Autodesk Inventor part; units mm, degrees
ref_plane "YZ Plane" through (0, 0, 0) normal (1, 0, 0) x (0, 1, 0)
ref_plane "XZ Plane" through (0, 0, 0) normal (0, 1, 0) x (-1, 0, 0)
ref_plane "XY Plane" through (0, 0, 0) normal (0, 0, 1) x (1, 0, 0)
sketch "Sketch1" plane through (0, 0, 0) normal (0, 1, 0) x (-1, 0, 0)
  line L0 (-6.7, 6.25) -> (6.7, 6.25)
  line L1 (6.7, 6.25) -> (6.7, -6.25)
  line L2 (6.7, -6.25) -> (-6.7, -6.25)
  line L3 (-6.7, -6.25) -> (-6.7, 6.25)
  line L4 (-6.7, 6.25) -> (6.7, -6.25) construction
  line L5 (6.7, 6.25) -> (-6.7, -6.25) construction
  point P0 (0, 0)
  dimension "d0" = 13.4
  dimension "d1" = 12.5
extrude "Extrusion1" add sketch "Sketch1" along normal blind 6.5
sketch "Sketch2" plane through (0, 6.5, 0) normal (0, 1, 0) x (1, 0, 0)
  circle A0 centre (0, 0) radius 3.5
  dimension "d4" = 7
extrude "Extrusion2" add sketch "Sketch2" along normal blind 5
sketch "Sketch3" plane through (0, 11.5, 0) normal (0, 1, 0) x (1, 0, 0)
  circle A0 centre (0, 0) radius 3
  dimension "d7" = 6
extrude "Extrusion3" add sketch "Sketch3" along normal blind 10
sketch "Sketch4" plane through (0, 21.5, 0) normal (0, 1, 0) x (1, 0, 0)
  line L0 (0, -1.5) -> (2.5981, -1.5)
  circle A0 centre (0, 0) radius 3
  line L1 (0, -1.5) -> (-2.5981, -1.5)
  arc A1 (-2.5981, -1.5) -> (2.5981, -1.5) centre (0, 0) ccw
  dimension "d10" = 1.5
extrude "Extrusion4" cut sketch "Sketch4" against normal blind 7 contours L0 A0 L1 picked at (-1.5934, -1.6862)
thread "Thread1"
properties part number "PEC11R-4215F-S0024"
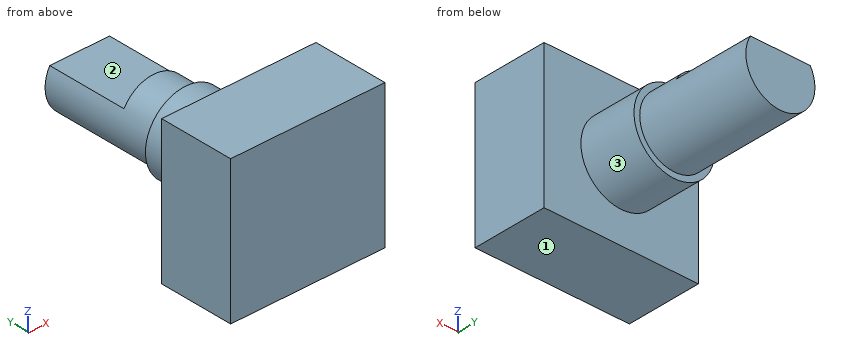
Input: part model. Units: mm. Frame: model coordinates. Face numbers are marked on the shaded views. A direction names the side the tool comes from. Give positions to 0.01 mm unless a question says otherwise; leave off trailing zeros. Loops run counter-clockwise (first coordinate to the right, second up) from the corner with the lowest first, then second, coordinate; pieces in that order, holes last.
1) Contact query for flat-ended pins moving along their axis: pin 1 (5.5 mm diameter, centred on x = 0, y = 17, fed in from +Z); pin 2 (0.5 mm diameter, centred on x = -1, z = 2, fed in from +Y); pin 3 (3 mm diameter, centred on x = -5, y = 12.5, fed in from +Z); pin 4 (1.5 mm diameter, centred on y = 12.5, z = 1, fed in from -X). Output: stop coordinate, or through.
A:
pin 1: stops at z = 3
pin 2: stops at y = 14.5
pin 3: passes through
pin 4: stops at x = -2.99
2) Section query B-B on z = 0. Return the cut outline in (x, y), and give its area (3 significant figures).
A:
outline: (-6.7, 0) - (6.7, 0) - (6.7, 6.5) - (3.5, 6.5) - (3.5, 11.5) - (3, 11.5) - (3, 21.5) - (-3, 21.5) - (-3, 11.5) - (-3.5, 11.5) - (-3.5, 6.5) - (-6.7, 6.5) - close
area: 182 mm2
3) Section query D-D on z = 2.25. Return the cut outline in (x, y), and give its area (3 significant figures).
A:
outline: (-6.7, 0) - (6.7, 0) - (6.7, 6.5) - (2.68, 6.5) - (2.68, 11.5) - (1.98, 11.5) - (1.98, 14.5) - (-1.98, 14.5) - (-1.98, 11.5) - (-2.68, 11.5) - (-2.68, 6.5) - (-6.7, 6.5) - close
area: 126 mm2
4) Section query C-C on y = 13. Return the cut outline in (x, z).
A:
outline: circle Ø6 at (0, 0)
5) Reachability of the marked faces 1, 2 and 3 from +Z, -Z, +X, -X, +Y, -Y: full face, straight path, thin tool, end or side. Return the list, or none.
A:
face 1: -Z, +X, -X, +Y, -Y
face 2: +Z, +X, -X, +Y
face 3: +Y
6) Section query A-A on x = 0. Return the cut outline in (y, z).
A:
outline: (0, -6.25) - (6.5, -6.25) - (6.5, -3.5) - (11.5, -3.5) - (11.5, -3) - (21.5, -3) - (21.5, 1.5) - (14.5, 1.5) - (14.5, 3) - (11.5, 3) - (11.5, 3.5) - (6.5, 3.5) - (6.5, 6.25) - (0, 6.25) - close
7) Line query: L1, parallel to Y at x = 5.25, z = -1; L2, parallel to X at y = 8, z = -2.5; L3, parallel to Z at x = -2.25, y = 9.75. Output: solid intervals per line, ascending.
A:
L1: y = 0 to 6.5
L2: x = -2.45 to 2.45
L3: z = -2.68 to 2.68
